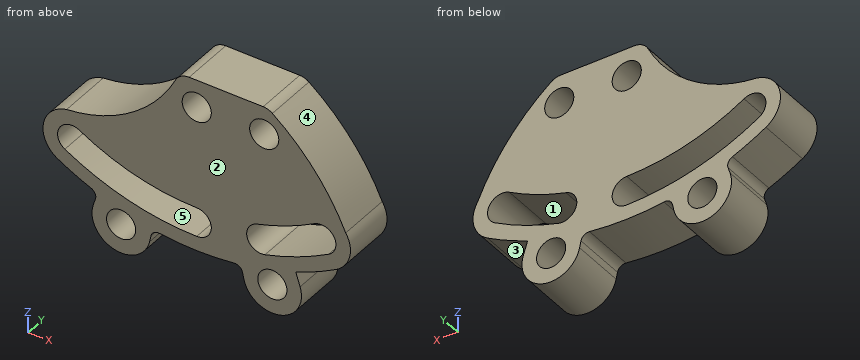
from build123d import *

# Parameters (mm, degrees)
SKETCH2_R           = 4.826
BOSS_EXTRUDE1_DEPTH = 17.78


with BuildPart() as part:
    # Sketch2 → Boss-Extrude1 (new body)
    with BuildSketch(Plane(origin=(0, 0, 0), x_dir=(1, 0, 0), z_dir=(0, 1, 0))):
        with BuildLine():
            ThreePointArc((15.610859978, 51.056586824), (27.545075694, 58.349621989), (34.233892096, 46.066560407))
            Line((34.233892096, 46.066560407), (32.812957113, 41.715646574))
            ThreePointArc((32.812957113, 41.715646574), (39.58316936, 38.822933823), (46.101, 35.39927428))
            ThreePointArc((46.101, 35.39927428), (50.667182056, 29.264811664), (49.337445304, 21.733978355))
            ThreePointArc((49.337445304, 21.733978355), (39.143444972, 4.93100158), (25.060604801, -8.777801578))
            ThreePointArc((25.060604801, -8.777801578), (23.616284404, -9.536863302), (22.005826143, -9.798894416))
            Line((22.005826143, -9.798894416), (-2.51457971, -9.798894416))
            ThreePointArc((-2.51457971, -9.798894416), (-5.192160007, -9.035949402), (-7.065470014, -6.976281719))
            ThreePointArc((-7.065470014, -6.976281719), (-21.858610455, 10.006362304), (-43.076963776, 17.558096172))
            ThreePointArc((-43.076963776, 17.558096172), (-50.791269491, 25.427412588), (-46.101, 35.39927428))
            ThreePointArc((-46.101, 35.39927428), (-40.648214467, 38.308271276), (-35.012800321, 40.845443124))
            ThreePointArc((-35.012800321, 40.845443124), (-33.673672112, 42.125267238), (-33.559725058, 43.974112877))
            Line((-33.559725058, 43.974112877), (-34.233892096, 46.066560407))
            ThreePointArc((-34.233892096, 46.066560407), (-27.545075694, 58.349621989), (-15.610859978, 51.056586824))
            Line((-15.610859978, 51.056586824), (-15.148481995, 48.907390587))
            ThreePointArc((-15.148481995, 48.907390587), (-14.125378132, 47.363216824), (-12.325747026, 46.924420733))
            ThreePointArc((-12.325747026, 46.924420733), (0, 47.752), (12.325747026, 46.924420733))
            ThreePointArc((12.325747026, 46.924420733), (14.125378132, 47.363216824), (15.148481995, 48.907390587))
            Line((15.148481995, 48.907390587), (15.610859978, 51.056586824))
        make_face()
        with Locations(Location((0, -0.668228959, 0), (0, 0, 270))):
            Circle(SKETCH2_R, mode=Mode.SUBTRACT)
        with Locations(Location((22.352, -0.668228959, 0), (0, 0, 270))):
            Circle(SKETCH2_R, mode=Mode.SUBTRACT)
        with Locations(Location((-25.046954271, 49.026505913, 0), (0, 0, 270))):
            Circle(SKETCH2_R, mode=Mode.SUBTRACT)
        with Locations(Location((25.046954271, 49.026505913, 0), (0, 0, 270))):
            Circle(SKETCH2_R, mode=Mode.SUBTRACT)
        with BuildLine():
            ThreePointArc((-43.688, 31.219835681), (-45.454438599, 24.627397082), (-38.862, 22.860958484))
            ThreePointArc((-38.862, 22.860958484), (-20.116451462, 30.625618922), (0, 33.274))
            ThreePointArc((0, 33.274), (4.826, 38.1), (0, 42.926))
            ThreePointArc((0, 42.926), (-22.614572885, 39.948734998), (-43.688, 31.219835681))
        make_face(mode=Mode.SUBTRACT)
        with BuildLine():
            ThreePointArc((22.614572885, 39.948734998), (16.703954136, 36.536237672), (20.116451462, 30.625618922))
            ThreePointArc((20.116451462, 30.625618922), (29.743687097, 27.357612785), (38.862, 22.860958484))
            ThreePointArc((38.862, 22.860958484), (45.454438599, 24.627397082), (43.688, 31.219835681))
            ThreePointArc((43.688, 31.219835681), (33.437347586, 36.274898033), (22.614572885, 39.948734998))
        make_face(mode=Mode.SUBTRACT)
    extrude(amount=BOSS_EXTRUDE1_DEPTH)


solid = part.part
Source: CAD feature listing. Evaluate the final solid. Frame: model axes, mm. Face numbers are marked on the shaded views. A direction names the side the tool comes from. Round coordinates to 2 decimals unless told otherwise and drop trailing zeros. Loops run counter-clockwise (first coordinate to the right, second up) from the corner with the lowest first, then second, coordinate; pieces in that order, holes last. Notation, with made-up numbers: (-13.5, 5) - (-7.5, 5) arc R21 cw to (-7.5, 14) - close; hole circle Ø1 at (-36.75, 10). An arc over 180 degrees is marked (long way). Write item = value, one per line. Start each with the question number.
Item 1: Reachability of the marked faces 4 and 5 from +Z, -Z, +X, -X, +Y, -Y: full face, straight path, thin tool, end or side. Return the list, or none.
Item 2: Section query C-C on y = 14. Count the separate pieces of the cut face and the enclosed holes in it, plus the area to 3 significant figures.
Item 3: Material intervals for line 1 (X direction, y = 10.75, z = -49); line 2 (Z direction, x = 25, y = 7.25); line 3 (X direction, y = 11.5, z = -50.5), sorted ascending.
Item 4: First-contact query: pin 1 Ø3 at (y, z) = (3.5, -3.5) entering from +X; pin 2 Ø2 at (x, y) = (31, 13) entering from -Z; pin 3 Ø10 at (y, z) = (5, -44) entering from -X. Flat tips, straight axial feed; report the tip coordinate or a pass-through.
Item 5: Mould query, pull axis X, two halves, no side actions, for the marked faces 1, 2 and 3. Classes: released by +X, released by -X, zero draft, split by the parting line, or undercut.
Item 6: Section query D-D on x = -10. Output: boundary loops of the cut face in (y, z).
Item 7: Section query B-B on x = -40. Output: boundary loops of the cut face in (y, z) (3 decimals), plus the area to 3 significant figures.
Item 8: Section query A-A on z = -36.5. Output: boundary loops of the cut face in (x, y).
Results list:
q1.face_4 = +Z, +X, +Y, -Y
q1.face_5 = +Y, -Y
q2.separate_pieces = 1
q2.enclosed_holes = 6
q2.area = 3,430 mm²
q3.line_1 = -34.7 to -29.87, -20.22 to -15.17, 15.17 to 20.22, 29.87 to 34.7
q3.line_2 = -58.68 to -53.85, -44.2 to -39.27, -29.14 to -3.37, 4.7 to 8.82
q3.line_3 = -34.59 to -29.64, -20.45 to -15.49, 15.49 to 20.45, 29.64 to 34.59
q4.pin_1 = 39.2
q4.pin_2 = -57.31
q4.pin_3 = -39.21
q5.face_1 = undercut
q5.face_2 = zero draft
q5.face_3 = released by +X
q6.outline = (0, -47.21) - (17.78, -47.21) - (17.78, -42.35) - (0, -42.35) - close; (0, -32.63) - (17.78, -32.63) - (17.78, 1.92) - (0, 1.92) - close
q7.outline = (0, -38.624) - (17.78, -38.624) - (17.78, -33.232) - (0, -33.232) - close; (0, -22.386) - (17.78, -22.386) - (17.78, -17.185) - (0, -17.185) - close
q7.area = 188 mm²
q8.outline = (-44.14, 0) - (-32.89, 0) - (-32.89, 17.78) - (-44.14, 17.78) - close; (4.55, 0) - (16.69, 0) - (16.69, 17.78) - (4.55, 17.78) - close; (32.89, 0) - (44.14, 0) - (44.14, 17.78) - (32.89, 17.78) - close
